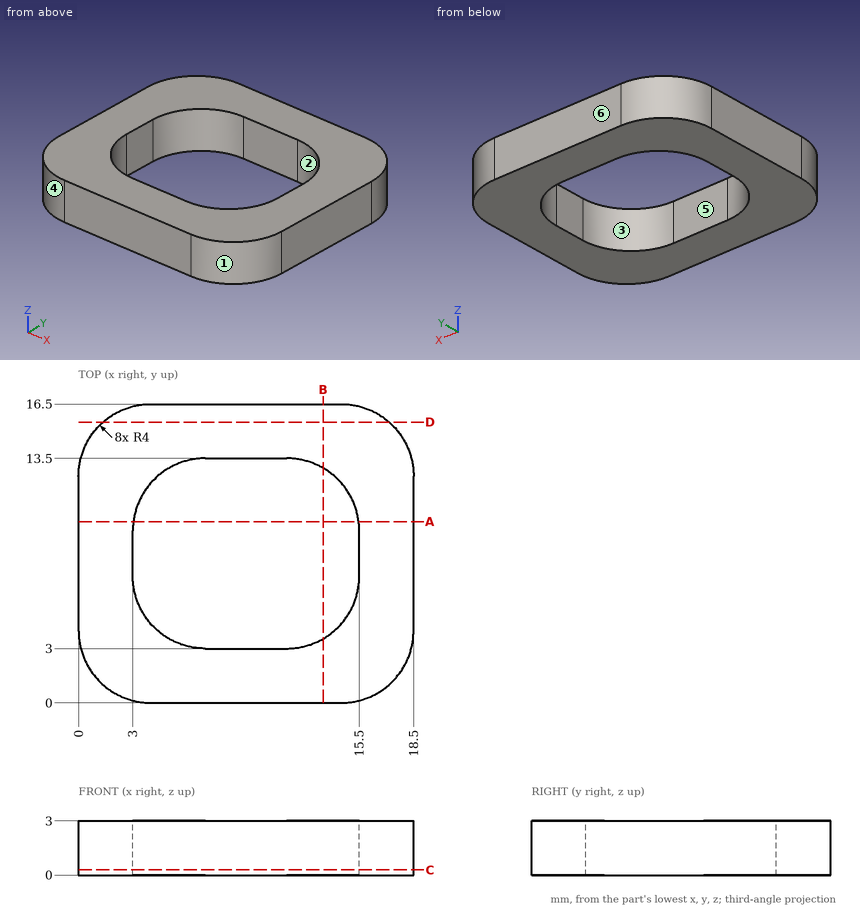
Geometry: see drawing. Coordinates: mm, zero at the bounding-box minimum. A direction names the side the tool comes from. Coordinates: 2 decimals unless noted, no trailing zeros. Loops run counter-clockwise (first coordinate to the right, second up) from the corner with the lowest first, then second, coordinate; pieces in that order, holes last. Notation, with made-up numbers: M 35,-39 L 89,-39 A33 ccw 89,-2 Z; hole C 75.5,27 d5. An arc over 180 degrees is marked long. Answer in a Markdown table with one row per item.
Q1. Section A-A on y = 10. Return the cut outline in (x, z), plus the area to 3 significant figures.
Answers below:
| item | result |
|---|---|
| outline | M 0,0 L 3.03,0 L 3.03,3 L 0,3 Z; M 15.47,0 L 18.5,0 L 18.5,3 L 15.47,3 Z |
| area | 18.2 mm^2 |
Q2. Ray query, probe 1 along X at (y, z) = (8.75, 1); probe 2 along Y at (x, z) = (8, 1.55); probe 3 along X at (y, z) = (10.5, 0.95). Return the intervals inside material, ascending. Write a range as from..to.
Answers below:
| item | result |
|---|---|
| probe 1 | x = 0..3, 15.5..18.5 |
| probe 2 | y = 0..3, 13.5..16.5 |
| probe 3 | x = 0..3.13, 15.37..18.5 |
Q3. Draft query along X for the marked faces 3, 4, 5 and 6. Return one class per face: pulls with the +X half, pulls with the -X half, needs draft (parallel to the pull), parting line crosses it, or undercut.
Answers below:
| item | result |
|---|---|
| face 3 | undercut |
| face 4 | pulls with the -X half |
| face 5 | undercut |
| face 6 | needs draft |
Q4. First-contact query: pin 1 (1 mm diameter, centred on y = 11.5, z = 1.5, fed in from -X); pin 2 (1.5 mm diameter, centred on x = 11.5, y = 12.5, fed in from +Z). Flat tips, straight axial feed; report the tip coordinate or a pass-through.
Answers below:
| item | result |
|---|---|
| pin 1 | stops at x = 0 |
| pin 2 | passes through |
Q5. Section D-D on y = 15.5. Return the cut outline in (x, z).
Answers below:
| item | result |
|---|---|
| outline | M 1.35,0 L 17.15,0 L 17.15,3 L 1.35,3 Z |
Q6. Section C-C on z = 0.3. Return the cut outline in (x, y), plus the area to 3 significant figures.
Answers below:
| item | result |
|---|---|
| outline | M 0,4 A4 ccw 4,0 L 14.5,0 A4 ccw 18.5,4 L 18.5,12.5 A4 ccw 14.5,16.5 L 4,16.5 A4 ccw 0,12.5 Z; hole M 3,7 A4 ccw 7,3 L 11.5,3 A4 ccw 15.5,7 L 15.5,9.5 A4 ccw 11.5,13.5 L 7,13.5 A4 ccw 3,9.5 Z |
| area | 174 mm^2 |
Q7. Section B-B on x = 13.5. Return the cut outline in (y, z).
Answers below:
| item | result |
|---|---|
| outline | M 0,0 L 3.54,0 L 3.54,3 L 0,3 Z; M 12.96,0 L 16.5,0 L 16.5,3 L 12.96,3 Z |
Q8. Set-up query: the marked faces 1 and 2. Return all of +Z, -Z, +X, -X, +Y, -Y with unobstructed straight access to the full face (end or side cutting, diameter ignored); none if empty.
Answers below:
| item | result |
|---|---|
| face 1 | +Z, -Z, +X, -Y |
| face 2 | +Z, -Z |
